```python
from build123d import *

# Parameters (mm, degrees)
SKETCH_OF_SERVO_MOTOR_W               = 42.5
SKETCH_OF_SERVO_MOTOR_H               = 54
EXTRUDE_BASE_OF_FOOT_DEPTH            = 5
POSITIONS_OF_FOOT_SIDES_W             = 5
POSITIONS_OF_FOOT_SIDES_H             = 54
POSITIONS_OF_FOOT_SIDES_H_2           = 6.8
EXTRUDE_SIDES_OF_FOOT_DEPTH           = 19
FILLET_TOP_EDGES_OF_SIDES_OF_FOOT_R   = 3.5
EXTRUDE_FOOT_LIPS_DEPTH               = 42.5
FILLET_FOOT_LIPS_R                    = 4.1
HOLE_DIMENSIONS_FOR_M4_BOLT_R         = 2
EXTRUDE_CUT_HOLE_FOR_M4_BOLT_DEPTH    = 5
CUT_EXTRUDE1_REACH                    = 77.278
DIMENSIONS_FOR_OUTSIDE_FOOT_M4_HOLE_R = 2


with BuildPart() as part:
    # Sketch of Servo Motor → Extrude Base of Foot (new body)
    with BuildSketch(Plane(origin=(0, 0, 0), x_dir=(1, 0, 0), z_dir=(0, 1, 0))):
        with Locations((10.65, -20.2)):
            Rectangle(SKETCH_OF_SERVO_MOTOR_W, SKETCH_OF_SERVO_MOTOR_H)
    extrude(amount=-EXTRUDE_BASE_OF_FOOT_DEPTH)

    # Positions of Foot Sides → Extrude Sides of Foot (add)
    with BuildSketch(Plane(origin=(0, 0, 0), x_dir=(1, 0, 0), z_dir=(0, 1, 0))):
        with Locations((29.4, -20.2)):
            Rectangle(POSITIONS_OF_FOOT_SIDES_W, POSITIONS_OF_FOOT_SIDES_H)
        with Locations((2.5, 3.4)):
            Rectangle(POSITIONS_OF_FOOT_SIDES_W, POSITIONS_OF_FOOT_SIDES_H_2)
        with Locations((2.5, -43.8)):
            Rectangle(POSITIONS_OF_FOOT_SIDES_W, POSITIONS_OF_FOOT_SIDES_H_2)
    extrude(amount=EXTRUDE_SIDES_OF_FOOT_DEPTH)

    # Fillet Top Edges of Sides of Foot
    fillet_top_edges_of_sides_of_foot_edges = [part.edges().sort_by_distance(p)[0] for p in [
        (2.5, 19, -6.8),
        (2.5, 19, 47.2),
        (29.4, 19, -6.8),
        (29.4, 19, 47.2),
    ]]
    fillet(fillet_top_edges_of_sides_of_foot_edges, radius=FILLET_TOP_EDGES_OF_SIDES_OF_FOOT_R)

    # Front and Back Foot Lips → Extrude Foot Lips (add, through all)
    with BuildSketch(Plane.ZY.offset(10.6)):
        Polygon((60.767406064, 4.5), (58.418174512, 7.855050358), (47.2, 0), (47.2, -5), align=None)
        Polygon((-6.8, 0), (-6.8, -5), (-20.367406064, 4.5), (-18.018174512, 7.855050358), align=None)
    extrude(amount=-EXTRUDE_FOOT_LIPS_DEPTH)

    # Fillet Foot Lips
    # the kernel refuses this fillet: 4.1 mm, written as the material it takes off along each edge
    with BuildSketch(Plane(origin=(-20.85, 4.5, 60.767406064), x_dir=(0, 0.8191520442889908, -0.5735764363510476), z_dir=(1, 0, 0)), Plane(origin=(-20.85, 4.5, -20.367406064), x_dir=(0, -0.5735764363510438, 0.8191520442889934), z_dir=(1, 0, 0))) as fillet_foot_lips_piece_1:
        with BuildLine():
            CenterArc((FILLET_FOOT_LIPS_R, -FILLET_FOOT_LIPS_R), FILLET_FOOT_LIPS_R, 90, 90)
            Line((0, -FILLET_FOOT_LIPS_R), (0, 0))
            Line((0, 0), (FILLET_FOOT_LIPS_R, 0))
        make_face()
    extrude(amount=63, mode=Mode.SUBTRACT)

    # Hole Dimensions for M4 Bolt → Extrude Cut Hole for M4 Bolt (cut)
    with BuildSketch(Plane.ZY):
        with Locations((-3.324953132, 14.258904835)):
            Circle(HOLE_DIMENSIONS_FOR_M4_BOLT_R)
        with Locations((-3.377058396, 4.358904835)):
            Circle(HOLE_DIMENSIONS_FOR_M4_BOLT_R)
        with Locations((43.724953132, 14.258904835)):
            Circle(HOLE_DIMENSIONS_FOR_M4_BOLT_R)
        with Locations((43.777058396, 4.358904835)):
            Circle(HOLE_DIMENSIONS_FOR_M4_BOLT_R)
    extrude(amount=-EXTRUDE_CUT_HOLE_FOR_M4_BOLT_DEPTH, mode=Mode.SUBTRACT)

    # Dimensions for Outside Foot M4 Hole → Cut-Extrude1 (cut, up to next)
    with BuildSketch(Plane(origin=(31.9, 0, 0), x_dir=(0, 0, -1), z_dir=(1, 0, 0)), mode=Mode.PRIVATE) as cut_extrude1_sk1:
        with Locations((-29.2, 7)):
            Circle(DIMENSIONS_FOR_OUTSIDE_FOOT_M4_HOLE_R)
    cut_extrude1_tool1 = extrude(cut_extrude1_sk1.sketch, amount=-CUT_EXTRUDE1_REACH, mode=Mode.PRIVATE) & part.part
    add(cut_extrude1_tool1.solids().sort_by_distance((31.9, 7, 29.2))[0], mode=Mode.SUBTRACT)


solid = part.part
```
Geometry: final body of the model. Coordinates: model frame, mm. A direction names the side the tool comes from. Give positions to 0.01 mm unless a question says otherwise; leave off trailing zeros. Loops run counter-clockwise (first coordinate to the right, second up) from the corner with the lowest first, then second, coordinate; pieces in that order, holes last. Notation, with made-up numbers: (-31, 81) -> (-23, 81) arc R23 cw to (-23, 109) -> close; hole circle Ø5 at (20.25, -25.75). An arc over 180 degrees is marked (long way). Use CSV: the item, a comma, the result in double quotes.
(1) Access query for faces 1 (the face through (2.465, 4.96, 45.685)), 2 (the face through (5, 9, 44)), 3 (the face through (10, -5, 20)), 4 (the face through (2, 8, -6.8)). Directions: +Z, -Z, +X, -X, +Y, -Y. A direction counts if a zero-diameter tool reaches every point of the face in a straight line with its end or side. Return the directions, or none.
From the geometry:
face 1,"-X"
face 2,"+Y"
face 3,"+Z, -Z, +X, -X, -Y"
face 4,"+X, -X, +Y"
(2) Pull-direction query (Z, two-part tool) for faces 5 (the face through (29.435, 7.088, 31.198)), 6 (the face through (5, 9, -3)), 7 (the face through (2.54, 18, 46.15)), 8 (the face through (-10.6, -2, 20)); classes: released by +Z, released by -Z, zero draft, split by the parting line, or undercut.
From the geometry:
face 5,"undercut"
face 6,"undercut"
face 7,"released by +Z"
face 8,"zero draft"
(3) First-contact query: P1, Ø2, axis at y = 6.5, z = 44.5, coming from the -X side; P2, Ø4, axis at x = 1.5, y = 12.5, coming from the +Z side; P3, Ø2.5, axis at x = 3.5, y = 8.5, coming from the -Z side. Flat tips, straight axial feed; report the tip coordinate or a pass-through.
From the geometry:
P1,"x = 0"
P2,"z = 47.2"
P3,"z = -18.37"
(4) Ray query, line 1 along Z through (x, y) = (2, 14.5); line 2 along X through (y, z) = (17.25, -1.5); line 3 along Z through (x, y) = (29, 4.5). Return the intervals inside material, ascending. Write a range as [from, to].
From the geometry:
line 1,"[-6.8, -5.31], [-1.34, 0], [40.4, 41.74], [45.71, 47.2]"
line 2,"[0, 5], [26.9, 31.9]"
line 3,"[-18.63, -13.23], [-6.8, 47.2], [53.63, 59.03]"
(5) Cut plane C-C (y = -1.5). Output: boundary loops of the cut face in (x, z), plus the area to 3 significant figures.
From the geometry:
outline,"(-10.6, -11.8) -> (31.9, -11.8) -> (31.9, 52.2) -> (-10.6, 52.2) -> close"
area,"2,720 mm^2"
(6) Cut plane B-B (x = 8.5). Output: boundary loops of the cut face in (y, z), plus the area to 3 significant figures.
From the geometry:
outline,"(-5, -6.8) -> (2.15, -17.01) arc R4.1 ccw to (7.86, -18.02) -> (0, -6.8) -> (0, 47.2) -> (7.86, 58.42) arc R4.1 ccw to (2.15, 57.41) -> (-5, 47.2) -> close"
area,"387 mm^2"
(7) Cut plane A-A (z = 29.2). Output: boundary loops of the cut face in (x, y), plus the area to 4 significant figures.
From the geometry:
outline,"(-10.6, -5) -> (31.9, -5) -> (31.9, 5) -> (26.9, 5) -> (26.9, 0) -> (-10.6, 0) -> close; (26.9, 9) -> (31.9, 9) -> (31.9, 19) -> (26.9, 19) -> close"
area,"287.5 mm^2"
